Input: dimensioned drawing with shaded views. Units: mm. Origin: part minimum x, y, z. A direction names the side the tool comes from. Give positions to 0.01 mm unless a question says otherwise; leave off trailing zeros. Order: outer loops, then holes, each group sorted by start corner. A loop starts at its lowest first (then second) coordinate and runs counter-clockwise, first axis right, second up. Notation, with made-up numbers: (47.25, -7) - (56.25, -7) arc R32 cw to (56.25, 32) - close; hole circle Ø8 at (69.25, 21.25). An arc over 180 degrees is marked (long way). Use a Markdown table: item, result.
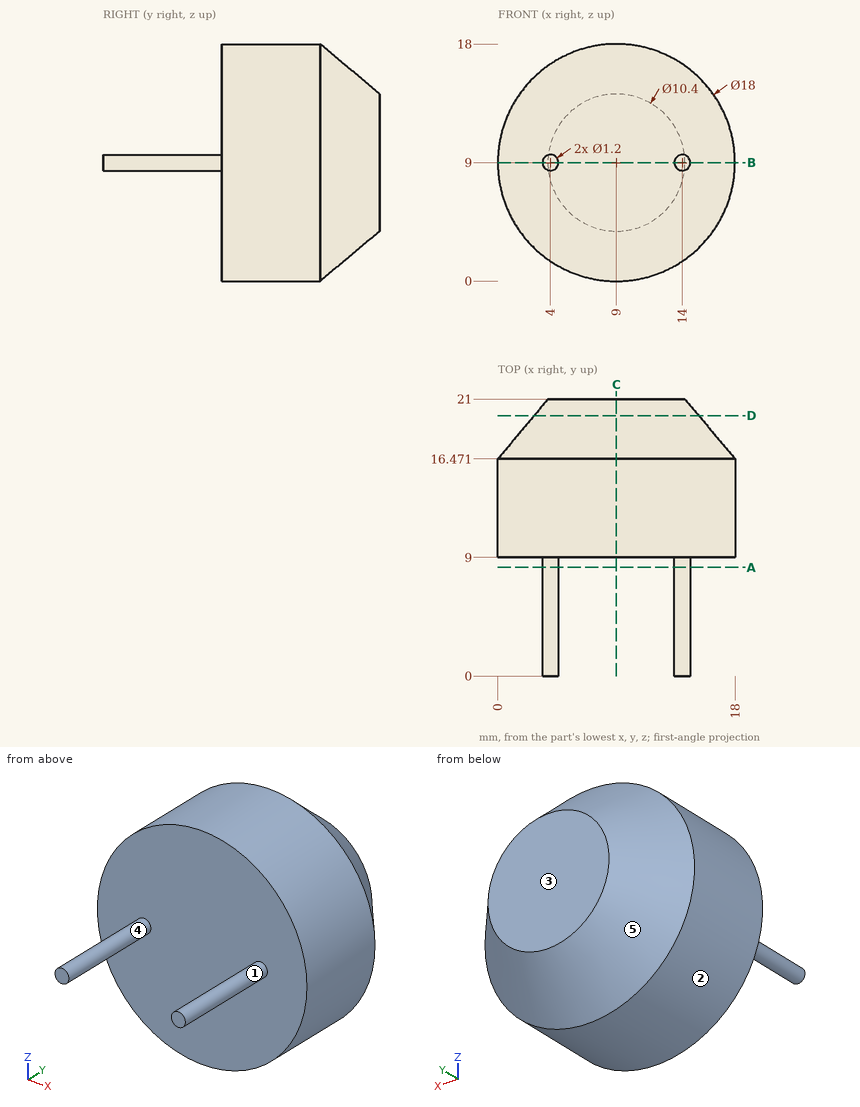
1. Mould query, pull axis X, two halves, no side actions, for the marked faces 1, 2 and 3. Classes: pulls with the +X half, pulls with the -X half, needs draft (parallel to the pull), parting line crosses it, or undercut.
Response:
| item | result |
|---|---|
| face 1 | undercut |
| face 2 | parting line crosses it |
| face 3 | needs draft |
2. Section query D-D (y = 19.75). Return loops of the section in (x, z).
Response:
| item | result |
|---|---|
| outline | circle Ø12.5 at (9, 9) |
3. Section query C-C (x = 9). Return loops of the section in (y, z).
Response:
| item | result |
|---|---|
| outline | (9, 0) - (16.47, 0) - (21, 3.8) - (21, 14.2) - (16.47, 18) - (9, 18) - close |
4. Section query B-B (z = 9). Return loops of the section in (x, y), then the cut area to 3 significant figures.
Response:
| item | result |
|---|---|
| outline | (0, 9) - (3.4, 9) - (3.4, 0) - (4.6, 0) - (4.6, 9) - (13.4, 9) - (13.4, 0) - (14.6, 0) - (14.6, 9) - (18, 9) - (18, 16.47) - (14.2, 21) - (3.8, 21) - (0, 16.47) - close |
| area | 220 mm^2 |
5. Section query A-A (y = 8.25). Return loops of the section in (x, z).
Response:
| item | result |
|---|---|
| outline | circle Ø1.2 at (4, 9); circle Ø1.2 at (14, 9) |
6. Material intervals for line 1 along Y through (x, z) = (9.25, 4.25); line 2 along Z through (x, y) = (4, 4.75); line 3 along Z through (x, y) = (12, 13.5) (1 decimal), sorted ascending.
Response:
| item | result |
|---|---|
| line 1 | y = 9 to 21 |
| line 2 | z = 8.4 to 9.6 |
| line 3 | z = 0.5 to 17.5 |
7. Set-up query: the marked faces 4 and 5. Return all of +Z, -Z, +X, -X, +Y, -Y with unobstructed straight access to the full face (end or side cutting, diameter ignored); none if empty.
Response:
| item | result |
|---|---|
| face 4 | -Y |
| face 5 | +Y |
8. Pin query (flat end, axial travel): pin 1 (1.5 mm diameter, centred on x = 10, z = 15.5, fed in from -Y); pin 2 (8 mm diameter, centred on x = 14.5, y = 9, fed in from +Z); pin 3 (3 mm diameter, centred on y = 8, z = 3.5, fed in from -X). Return the tip coordinate at first contact, or that it passes through.
Response:
| item | result |
|---|---|
| pin 1 | stops at y = 9 |
| pin 2 | stops at z = 17.87 |
| pin 3 | stops at x = 1.14 |
